from build123d import *

# Parameters (mm, degrees)
F0_R      = 14.605
F1_DEPTH  = 12.7
F2_R      = 6.35
F3_DEPTH  = 30.48
F5_DEPTH  = 38.1
F6_R      = 8.255
F7_DEPTH  = 2.3
F8_R      = 5.06
F9_DEPTH  = 4.1
F11_D     = 3.1
F12_R     = 0.762
F13_R     = 4
F14_DEPTH = 33.02
F20_D     = 2.2606
F20_DEPTH = 12.7
F20_START = 0.0438035
F20_TIP   = 0.6791527577


with BuildPart() as f1:
    # F0 (on Top) → F1 (new body)
    with BuildSketch(Plane.XY):
        Circle(F0_R)
    extrude(amount=F1_DEPTH)

    # F2 (on face) → F3 (join)
    with BuildSketch(Plane.XY.offset(12.7)):
        Circle(F2_R)
    extrude(amount=F3_DEPTH)

    # F4 (on face) → F5 (join)
    with BuildSketch(Plane.XY.offset(43.18)):
        Polygon((2.7276336118, -4.7244), (5.4552672235, 0), (2.7276336118, 4.7244), (-2.7276336118, 4.7244), (-5.4552672235, 0), (-2.7276336118, -4.7244), align=None)
    extrude(amount=F5_DEPTH)

    # F6 (on face) → F7 (cut)
    with BuildSketch(Plane(origin=(0, 0, 0), x_dir=(1, 0, 0), z_dir=(0, 0, -1))):
        Circle(F6_R)
    extrude(amount=-F7_DEPTH, mode=Mode.SUBTRACT)

    # F8 (on face) → F9 (cut)
    with BuildSketch(Plane(origin=(0, 0, 0), x_dir=(1, 0, 0), z_dir=(0, 0, -1))):
        Circle(F8_R)
    extrude(amount=-F9_DEPTH, mode=Mode.SUBTRACT)

    # F11 (through all)
    with Locations(Plane.XY.offset(12.7)):
        with Locations((0, -10.05), (-10.05, 0), (0, 10.05), (10.05, 0)):
            Hole(F11_D / 2)

    # F12
    f12_edges = [f1.edges().sort_by_distance(p)[0] for p in [
        (-2.727634, -4.7244, 62.23),
        (2.727634, -4.7244, 62.23),
        (5.455267, 0, 62.23),
        (2.727634, 4.7244, 62.23),
        (-2.727634, 4.7244, 62.23),
        (-5.455267, 0, 62.23),
    ]]
    fillet(f12_edges, radius=F12_R)

    # F13 (on face) → F14 (cut)
    with BuildSketch(Plane(origin=(0, 0, 0), x_dir=(1, 0, 0), z_dir=(0, 0, -1))):
        Circle(F13_R)
    extrude(amount=-F14_DEPTH, mode=Mode.SUBTRACT)

    # F20
    # its depths count from where the whole tool has entered the part; down to there all is cleared
    with Locations(Plane(origin=(-10.3272945392, -10.3272945392, 0), x_dir=(-0.7071067812, 0.7071067812, 0), z_dir=(-0.7071067812, -0.7071067812, 0)).offset(-F20_START)):
        with Locations((0, -7.62)):
            Hole(F20_D / 2, depth=F20_DEPTH)
            with Locations((0, 0, -(F20_DEPTH + F20_TIP / 2))):  # 118° drill point
                Cone(0, F20_D / 2, F20_TIP, mode=Mode.SUBTRACT)


solid = f1.part
Check sheet for the modelled part. Datum: model origin and axes. Units: mm. A direction names the side the tool comes from. Round coordinates to 2 decimals unless told otherwise and drop trailing zeros. Loops run counter-clockwise (first coordinate to the right, second up) from the corner with the lowest first, then second, coordinate; pieces in that order, holes last.
1. Set-up check for faces 5 (the flat face through (-4.075, 2.39, 61.963)), 6 (the flat face through (-1, 5, 43.18)), 7 (the cylindrical face through (7.874, -2.48, 1.134)): record each of +Z, -Z, +X, -X, +Y, -Y from which the full face is reachable in a straight line by a thin tool's end or side.
2. Scan lines: probe 1 along Y at (x, z) = (0, 0.75) (3 decimals); probe 2 along Y at (x, z) = (0, 3.4) (3 decimals); probe 3 along Y at (x, z) = (0, 12.75). Record each from-to range of solid material in increasing order.
3. Sectioned sample at C-C on x = 10.05. Record the boundary of the cut face in (y, z).
4. Sectioned sample at B-B on z = 17. Record the boundary of the cut face in (x, y).
5. Gauge pin test, flat ends, axial feed: pin 1 Ø15 at (x, y) = (0, 0) entering from -Z; pin 2 Ø5 at (x, z) = (-0.5, 58) entering from +Y; pin 3 Ø1.5 at (x, z) = (-3.5, 52) entering from +Y. Record the tip position at first contact, or that the pin passes through.
6. Sectioned sample at A-A on x = 0. Give the number of separate pieces and of enclosed holes in the cut face, and give its area (3 significant figures).
7. Mould release check, pull along X, two halves, no side actions. Record for faces 1 (the flat face through (-4.11, -2.33, 61.96)), 2 (the flat face through (4.075, -2.39, 61.963)), 3 (the cylindrical face through (8.572, 0.466, 6.261)), 4 (the flat face through (0, -4.724, 62)): released by +X, released by -X, zero draft, split by the parting line, or undercut.
Recorded:
1. face 5: +Z, -X, +Y
1. face 6: +Z
1. face 7: -Z
2. probe 1: y = -14.605 to -11.6, -8.5 to -8.255, 8.255 to 8.5, 11.6 to 14.605
2. probe 2: y = -14.605 to -11.6, -8.5 to -5.06, 5.06 to 8.5, 11.6 to 14.605
2. probe 3: y = -6.35 to -4, 4 to 6.35
3. outline: (-10.6, 0) - (-1.55, 0) - (-1.55, 12.7) - (-10.6, 12.7) - close; (1.55, 0) - (10.6, 0) - (10.6, 12.7) - (1.55, 12.7) - close
4. outline: circle Ø12.7 at (0, 0); hole circle Ø8 at (0, 0)
5. pin 1: stops at z = 2.3
5. pin 2: stops at y = 4.72
5. pin 3: stops at y = 4.57
6. separate pieces: 3
6. enclosed holes: 0
6. area: 752 mm2
7. face 1: released by -X
7. face 2: released by +X
7. face 3: undercut
7. face 4: zero draft
